from build123d import *

# Parameters (mm, degrees)
BOSS_EXTRUDE1_DEPTH = 9
SKETCH2_R           = 1.45
CUT_EXTRUDE1_DEPTH  = 77.43471479
CUT_EXTRUDE2_REACH  = 78.435
SKETCH4_R           = 13
SHELL10_OUTLINE_W   = 84
SHELL10_OUTLINE_H   = 116.25
SHELL10_OUTLINE_R   = 4.45
SHELL10_OUTLINE_R_2 = 16
SHELL10_DEPTH       = 6
SKETCH5_R           = 16
CUT_EXTRUDE3_DEPTH  = 3
CUT_EXTRUDE4_REACH  = 78.14
SKETCH6_R           = 5.25
SKETCH6_W           = 42
SKETCH6_H           = 54
BOSS_EXTRUDE2_START = -2
SKETCH7_R           = 1.45
BOSS_EXTRUDE2_DEPTH = 2


# Read off the part's stored shape, not the designer's step: Shell10
with BuildPart() as part:
    # Sketch1 → Boss-Extrude1 (new body)
    with BuildSketch(Plane(origin=(0, 0, 0), x_dir=(1, 0, 0), z_dir=(0, 1, 0))):
        with BuildLine():
            Line((-42, -61.125), (42, -61.125))
            ThreePointArc((42, -61.125), (44.121320344, -60.246320344), (45, -58.125))
            Line((45, -58.125), (45, 58.125))
            ThreePointArc((45, 58.125), (44.121320344, 60.246320344), (42, 61.125))
            Line((42, 61.125), (-42, 61.125))
            ThreePointArc((-42, 61.125), (-44.121320344, 60.246320344), (-45, 58.125))
            Line((-45, 58.125), (-45, -58.125))
            ThreePointArc((-45, -58.125), (-44.121320344, -60.246320344), (-42, -61.125))
        make_face()
    extrude(amount=BOSS_EXTRUDE1_DEPTH)

    # Sketch2 → Cut-Extrude1 (cut, through all)
    with BuildSketch(Plane.XZ):
        with Locations(Location((-35.959, -52.125, 0), (0, 0, 270))):
            Circle(SKETCH2_R)
        with Locations(Location((-35.959, 37.875, 0), (0, 0, 270))):
            Circle(SKETCH2_R)
    cut_extrude1 = extrude(amount=-CUT_EXTRUDE1_DEPTH, mode=Mode.SUBTRACT)

    # Sketch4 → Cut-Extrude2 (cut, up to next)
    with BuildSketch(Plane(origin=(0, 9, 0), x_dir=(1, 0, 0), z_dir=(0, 1, 0)), mode=Mode.PRIVATE) as cut_extrude2_sk1:
        with Locations(Location((24.934417701, 34, 0), (0, 0, 270))):
            Circle(SKETCH4_R)
    cut_extrude2_tool1 = extrude(cut_extrude2_sk1.sketch, amount=-CUT_EXTRUDE2_REACH, mode=Mode.PRIVATE) & part.part
    add(cut_extrude2_tool1.solids().sort_by_distance((24.934418, 9, -34))[0], mode=Mode.SUBTRACT)

    # Mirror3: Cut-Extrude1 across plane
    add(cut_extrude1.mirror(Plane(origin=(0, 0, 0), x_dir=(0, 0, 1), z_dir=(1, 0, 0))), mode=Mode.SUBTRACT)

    # Shell10 outline → Shell10 (cut)
    with BuildSketch(Plane(origin=(0, 0, 0), x_dir=(1, 0, 0), z_dir=(0, 1, 0))):
        Rectangle(SHELL10_OUTLINE_W, SHELL10_OUTLINE_H)
        with Locations((-35.959, -37.875)):
            Circle(SHELL10_OUTLINE_R, mode=Mode.SUBTRACT)
        with Locations((35.959, -37.875)):
            Circle(SHELL10_OUTLINE_R, mode=Mode.SUBTRACT)
        with Locations((-35.959, 52.125)):
            Circle(SHELL10_OUTLINE_R, mode=Mode.SUBTRACT)
        with Locations((24.934417701, 34)):
            Circle(SHELL10_OUTLINE_R_2, mode=Mode.SUBTRACT)
        with Locations((35.959, 52.125)):
            Circle(SHELL10_OUTLINE_R, mode=Mode.SUBTRACT)
    extrude(amount=SHELL10_DEPTH, mode=Mode.SUBTRACT)

    # Sketch5 → Cut-Extrude3 (cut)
    with BuildSketch(Plane.XZ):
        with Locations(Location((24.934417701, -34, 0), (0, 0, 90))):
            Circle(SKETCH5_R)
    extrude(amount=-CUT_EXTRUDE3_DEPTH, mode=Mode.SUBTRACT)

    # Sketch6 → Cut-Extrude4 (cut, up to next)
    with BuildSketch(Plane.XZ.offset(-6), mode=Mode.PRIVATE) as cut_extrude4_sk1:
        with Locations(Location((35.434417701, 24.375, 0), (0, 0, 270))):
            Circle(SKETCH6_R)
    cut_extrude4_tool1 = extrude(cut_extrude4_sk1.sketch, amount=-CUT_EXTRUDE4_REACH, mode=Mode.PRIVATE) & part.part
    # Sketch6 → Cut-Extrude4 (cut, up to next)
    with BuildSketch(Plane.XZ.offset(-6), mode=Mode.PRIVATE) as cut_extrude4_sk2:
        with Locations(Location((14.434417701, 24.375, 0), (0, 0, 270))):
            Circle(SKETCH6_R)
    cut_extrude4_tool2 = extrude(cut_extrude4_sk2.sketch, amount=-CUT_EXTRUDE4_REACH, mode=Mode.PRIVATE) & part.part
    # Sketch6 → Cut-Extrude4 (cut, up to next)
    with BuildSketch(Plane.XZ.offset(-6), mode=Mode.PRIVATE) as cut_extrude4_sk3:
        with Locations(Location((24.934417701, 10.875, 0), (0, 0, 270))):
            Circle(SKETCH6_R)
    cut_extrude4_tool3 = extrude(cut_extrude4_sk3.sketch, amount=-CUT_EXTRUDE4_REACH, mode=Mode.PRIVATE) & part.part
    # Sketch6 → Cut-Extrude4 (cut, up to next)
    with BuildSketch(Plane.XZ.offset(-6), mode=Mode.PRIVATE) as cut_extrude4_sk4:
        with Locations(Location((24.934417701, 37.875, 0), (0, 0, 270))):
            Circle(SKETCH6_R)
    cut_extrude4_tool4 = extrude(cut_extrude4_sk4.sketch, amount=-CUT_EXTRUDE4_REACH, mode=Mode.PRIVATE) & part.part
    # Sketch6 → Cut-Extrude4 (cut, up to next)
    with BuildSketch(Plane.XZ.offset(-6), mode=Mode.PRIVATE) as cut_extrude4_sk5:
        with Locations((-14.065582299, 0)):
            Rectangle(SKETCH6_W, SKETCH6_H)
    cut_extrude4_tool5 = extrude(cut_extrude4_sk5.sketch, amount=-CUT_EXTRUDE4_REACH, mode=Mode.PRIVATE) & part.part
    add(cut_extrude4_tool1.solids().sort_by_distance((35.434418, 6, 24.375))[0], mode=Mode.SUBTRACT)
    add(cut_extrude4_tool2.solids().sort_by_distance((14.434418, 6, 24.375))[0], mode=Mode.SUBTRACT)
    add(cut_extrude4_tool3.solids().sort_by_distance((24.934418, 6, 10.875))[0], mode=Mode.SUBTRACT)
    add(cut_extrude4_tool4.solids().sort_by_distance((24.934418, 6, 37.875))[0], mode=Mode.SUBTRACT)
    add(cut_extrude4_tool5.solids().sort_by_distance((-14.065582, 6, 0))[0], mode=Mode.SUBTRACT)

    # Sketch7 → Boss-Extrude2 (add)
    with BuildSketch(Plane(origin=(0, 9, 0), x_dir=(1, 0, 0), z_dir=(0, 1, 0)).offset(BOSS_EXTRUDE2_START)):
        with Locations(Location((-35.959, -37.875, 0), (0, 0, 90))):
            Circle(SKETCH7_R)
        with Locations(Location((-35.959, 52.125, 0), (0, 0, 90))):
            Circle(SKETCH7_R)
        with Locations(Location((35.959, 52.125, 0), (0, 0, 90))):
            Circle(SKETCH7_R)
        with Locations(Location((35.959, -37.875, 0), (0, 0, 90))):
            Circle(SKETCH7_R)
    extrude(amount=BOSS_EXTRUDE2_DEPTH)


solid = part.part
Work out the finished part from the listing and answer in its coordinate system (mm). A direction names the side the tool comes from. Coordinates: 2 decimals unless noted, no trailing zeros. Order: outer loops, then holes, each group sorted by start corner. A loop starts at its lowest first (then second) coordinate and runs counter-clockwise, first axis right, second up. Notation, with made-up numbers: (-30.5, 5.25) - (19.5, 5.25) arc R25 cw to (19.5, 37.25) - close; hole circle Ø1 at (-36.75, 84). An arc over 180 degrees is marked (long way). Put each result on its own line as item: value. Start each with the question number.
1) Find section C-C (y = 4.75). State how many separate pieces and enclosed holes the cut face has, plus the area to 3 significant figures.
2) For a pull along Z with two mould halves and no side action, classify faces 1 (the flat face through (1, 4, -61.125)), 2 (the flat face through (38, 0, -52)), 3 (the flat face through (9, 6, -1)) as released by +Z, released by -Z, zero draft, split by the parting line, or undercut.
3) Find the intervals of material crossed by line 1 (X direction, y = 5.5, z = 38); line 2 (X direction, y = 1.75, z = 43); line 3 (Z direction, x = -24, y = 1) (3 decimals), in increasing order. Write a range as from..to.
4) Find section D-D (z = -34). Give the vertices of the cut face in (x, y).
5) Find section A-A (z = 17.5). Give the vertices of the cut face in (x, y).
6) Find section B-B (x = -18). Give the vertices of the cut face in (y, z) (3 decimals).
7) Flat-ended cylindrical pins translate along their axes: pin 1 (9.5 mm diameter, centred on x = 24.93, z = 37.88, fed in from +Y); pin 2 (0.9 mm diameter, centred on x = 35.5, z = -51.5, fed in from -Y); pin 3 (12 mm diameter, centred on x = 24.93, z = 10.88, fed in from -Y). Find the tip coordinate at first contact, or state that the pin passes through.
8) For faces 4 (the flat face through (6.934, 7, 0)), 5 (the flat face through (-45, 4, -1)), 6 (the flat face through (36, 7, 38)), determine the directions among +Z, -Z, +X, -X, +Y, -Y from which every point of the face is accessible in a straight line to the end or side of a thin tool.
Results list:
1. separate pieces: 6
1. enclosed holes: 6
1. area: 1,730 mm^2
2. face 1: released by -Z
2. face 2: zero draft
2. face 3: undercut
3. line 1: x = -45..-42, -40.41..-37.4, -34.51..-31.51, 31.51..34.51, 37.4..40.41, 42..45
3. line 2: x = -45..-42, 42..45
3. line 3: z = -61.125..-58.125, 58.125..61.125
4. outline: (-45, 0) - (-42, 0) - (-42, 6) - (8.93, 6) - (8.93, 3) - (11.93, 3) - (11.93, 9) - (-45, 9) - close; (37.93, 3) - (40.93, 3) - (40.93, 6) - (42, 6) - (42, 0) - (45, 0) - (45, 9) - (37.93, 9) - close
5. outline: (-45, 0) - (-42, 0) - (-42, 6) - (-35.07, 6) - (-35.07, 9) - (-45, 9) - close; (6.93, 6) - (42, 6) - (42, 0) - (45, 0) - (45, 9) - (6.93, 9) - close
6. outline: (0, -61.125) - (9, -61.125) - (9, -27) - (6, -27) - (6, -58.125) - (0, -58.125) - close; (0, 58.125) - (6, 58.125) - (6, 27) - (9, 27) - (9, 61.125) - (0, 61.125) - close
7. pin 1: passes through
7. pin 2: stops at y = 7
7. pin 3: stops at y = 6
8. face 4: +Y, -Y
8. face 5: +Z, -Z, -X, +Y, -Y
8. face 6: -Y
